```python
from build123d import *
from build123d.topology import SkipClean

# Parameters (mm, degrees)
ESBO_O1_R                = 55
RESSALTO_EXTRUS_O1_DEPTH = 6
ESBO_O2_R                = 10
RESSALTO_EXTRUS_O2_DEPTH = 8
FILETE3_R                = 20
ESBO_O3_R                = 2.575
CORTE_EXTRUS_O1_DEPTH    = 79.192071209
PADR_OCIRCULAR1_COUNT    = 16
CORTE_EXTRUS_O2_DEPTH    = 79.192071209


with BuildPart() as part:
    # Esboço1 → Ressalto-extrusão1 (new body)
    with BuildSketch(Plane.XY):
        Circle(ESBO_O1_R)
    extrude(amount=RESSALTO_EXTRUS_O1_DEPTH)

    # Esboço2 → Ressalto-extrusão2 (add)
    with BuildSketch(Plane.XY.offset(6)):
        Circle(ESBO_O2_R)
        with BuildLine():
            Line((-2.24624687, 2.1), (2.24624687, 2.1))
            ThreePointArc((2.24624687, 2.1), (0, -3.075), (-2.24624687, 2.1))
        make_face(mode=Mode.SUBTRACT)
    extrude(amount=RESSALTO_EXTRUS_O2_DEPTH)

    # Filete3
    # the kernel refuses this fillet: 20 mm, written as the material it adds along each edge
    with BuildSketch(Plane(origin=(0, 0, 6), x_dir=(1, 0, 0), z_dir=(0, -1, 0))) as filete3_piece_1:
        with BuildLine():
            CenterArc((26, 20), FILETE3_R, 216.869897646, 53.130102354)
            Line((10, 8), (9.68, 7.76))
            ThreePointArc((9.68, 7.76), (9.6, 4), (9.6, 0))
            Line((9.6, 0), (10, -0.4))
            Line((10, -0.4), (26, -0.4))
            Line((26, -0.4), (26, 0))
        make_face()
    revolve(axis=Axis((0, 0, 6), (0, 0, 1)))

    # Esboço3 → Corte-extrusão1 (cut, through all)
    with BuildSketch(Plane.XY.offset(6)):
        with Locations((0, 48)):
            Circle(ESBO_O3_R)
    corte_extrus_o1 = extrude(amount=-CORTE_EXTRUS_O1_DEPTH, mode=Mode.SUBTRACT)

    # PadrãoCircular1: Corte-extrusão1 ×16 about axis
    padr_ocircular1_axis = Axis((0, 0, 0), (0, 0, 1))
    for i in range(1, PADR_OCIRCULAR1_COUNT):
        add(corte_extrus_o1.rotate(padr_ocircular1_axis, i * 360 / PADR_OCIRCULAR1_COUNT), mode=Mode.SUBTRACT)

    # Esboço4 → Corte-extrusão2 (cut, through all)
    with SkipClean():  # the faces are left unmerged after this step: merging them gives an invalid solid
        with BuildSketch(Plane.XY.offset(6)):
            with BuildLine():
                Line((2.24624687, 2.1), (-2.24624687, 2.1))
                ThreePointArc((-2.24624687, 2.1), (0, -3.075), (2.24624687, 2.1))
            make_face()
        extrude(amount=-CORTE_EXTRUS_O2_DEPTH, mode=Mode.SUBTRACT)
    add(part.part.scale(1), mode=Mode.REPLACE)  # the faces are merged on a copy


solid = part.part
```
Geometry: final body of the model. Coordinates: model frame, mm. Round coordinates to 2 decimals unless told otherwise and drop trailing zeros. Write each loop counter-clockwise with the first axis right and the second up, starting at its lowest first coordinate (ties: lowest second). Pieces come first, ordered by that corner, then holes. Notation, with made-up numbers: (38, 35.25) -> (63, 35.25) arc R25 cw to (63, 60.25) -> close; hole circle Ø3 at (78.5, 6.25). An arc over 180 degrees is marked (long way). Return JSON: item names as keys, results as strings.
Q1. Ray query, line 1 (Y direction, x = -44.5, z = 5.25); line 2 (Y direction, x = -35.5, z = 3); line 3 (X direction, y = 1, z = 5). Return the intervals inside material, ascending.
From the geometry:
{"line 1": "-32.32 to -20.94, -15.8 to 15.8, 20.94 to 32.32", "line 2": "-42.01 to -35.99, -31.89 to 31.89, 35.99 to 42.01", "line 3": "-54.99 to -50.37, -45.63 to -2.91, 2.91 to 45.63, 50.37 to 54.99"}
Q2. Section B-B on z = 1.25. Give the number of separate pieces and of enclosed holes in the cut face, and give its area (3 significant figures).
From the geometry:
{"separate pieces": "1", "enclosed holes": "17", "area": "9,140 mm2"}
Q3. Section C-C on y = -40.5. Return the cut outline in (x, z).
From the geometry:
{"outline": "(-37.21, 0) -> (37.21, 0) -> (37.21, 6) -> (-37.21, 6) -> close"}
Q4. Section D-D on z = 10.25. Return the cut outline in (x, y) (3 decimals).
From the geometry:
{"outline": "circle Ø27.347 at (0, 0); hole (-2.246, 2.1) arc R3.075 ccw (long way) to (2.246, 2.1) -> close"}
Q5. First-contact query: pin 1 Ø8 at (y, z) = (31, 6) entering from +X; pin 2 Ø4 at (x, y) = (33.94, 33.94) entering from +Z; pin 3 Ø1 at (x, y) = (29, 44) entering from +Z; pin 4 Ø3 at (y, z) = (7.5, 12.5) entering from -X. Flat tips, straight axial feed; report the tip coordinate or a pass-through.
From the geometry:
{"pin 1": "x = 47.92", "pin 2": "through", "pin 3": "z = 6", "pin 4": "x = -10.58"}
Q6. Mould query, pull axis Y, two halves, no side actions, for faces 1 (the cylindrical face through (-46.577, -19.656, 3.042)), 2 (the cylindrical face through (-11.923, -53.692, 2.958)), 3 (the flat face through (-0.1, 2.4, 14)). Classes: +Y half, -Y half, draft (parallel to the pull), parting line (faces both ways), or undercut.
From the geometry:
{"face 1": "undercut", "face 2": "parting line", "face 3": "draft"}
Q7. Section A-A on x = 0. Return the cut outline in (y, z) (3 decimals), and give its area (3 significant figures).
From the geometry:
{"outline": "(-55, 0) -> (-50.575, 0) -> (-50.575, 6) -> (-55, 6) -> close; (-45.425, 0) -> (-3.075, 0) -> (-3.075, 14) -> (-10, 14) arc R20 cw to (-26, 6) -> (-45.425, 6) -> close; (2.1, 0) -> (45.425, 0) -> (45.425, 6) -> (26, 6) arc R20 cw to (10, 14) -> (2.1, 14) -> close; (50.575, 0) -> (55, 0) -> (55, 6) -> (50.575, 6) -> close", "area": "763 mm2"}
